from build123d import *

# Parameters (mm, degrees)
CHAMFER1_SIZE = 0.508


with BuildPart() as part:
    # Sketch1 → Revolve1 (revolve)
    with BuildSketch(Plane(origin=(0, 0, 0), x_dir=(0, 0, -1), z_dir=(1, 0, 0)), mode=Mode.PRIVATE) as revolve1_sk:
        Polygon((-85.5345, 19.05), (88.4465, 19.05), (88.4465, 25), (86.4145, 25), (86.4145, 23.5), (84.2645, 23.5), (84.2645, 25), (-84.2645, 25), (-84.2645, 25.4), (-85.5345, 25.4), align=None)
    revolve(revolve1_sk.sketch.rotate(Axis((0, 0, 0), (0, 0, 1)), 90), axis=Axis((0, 0, 0), (0, 0, 1)))

    # Chamfer1
    chamfer1_edges = [part.edges().sort_by_distance(p)[0] for p in [
        (25, 0, -88.4465),
    ]]
    chamfer(chamfer1_edges, length=CHAMFER1_SIZE)


solid = part.part
Part model, mm, in its own coordinate system. A direction names the side the tool comes from. Coordinates: 2 decimals unless noted, no trailing zeros. Order: outer loops, then holes, each group sorted by start corner. A loop starts at its lowest first (then second) coordinate and runs counter-clockwise, first axis right, second up. Notation, with made-up numbers: (-13.5, 45) - (24.5, 45) arc R14 ccw to (24.5, 50) - close; hole circle Ø4 at (16.5, -24.5). An arc over 180 degrees is marked (long way). Use CSV: the item, a comma, the result in double quotes.
Item 1: Saw through at C-C on z = -44.5. Give the cut face in (x, y).
Solved:
outline,"circle Ø50 at (0, 0); hole circle Ø38.1 at (0, 0)"
Item 2: Probe probe 1 along Y at (x, z) = (0, -53.5); probe 2 along X at (y, z) = (1, 66); probe 3 along Y at (x, z) = (-7.5, 28.5). List the from-to ranges inside material, lowest first.
Solved:
probe 1,"y = -25 to -19.05, 19.05 to 25"
probe 2,"x = -24.98 to -19.02, 19.02 to 24.98"
probe 3,"y = -23.85 to -17.51, 17.51 to 23.85"
Item 3: Mould opens along Z. For faces 1 (the face through (-17, 17, -84.264)), 2 (the face through (4.13, 18.597, -2.674)), 3 (the face through (-4, -19, 85.534)) say: +Z half, -Z half, draft (parallel to the pull), parting line (faces both ways), or undercut.
Solved:
face 1,"undercut"
face 2,"draft"
face 3,"+Z half"
Item 4: Drop flat-ended pins along their axis: P1, Ø8, axis at x = -14, z = -38.5, coming from the -Y side; P2, Ø2, axis at y = 1.5, z = -49, coming from the +X side (3 decimals); P3, Ø10, axis at y = -20, z = -11.5, coming from the +X side. Give the stop position or say it passes through.
Solved:
P1,"stops at y = -22.91"
P2,"stops at x = 24.995"
P3,"stops at x = 20"
Item 5: Saw through at A-A on x = 0. Give the cut face in (y, z), and give its area (3 significant figures).
Solved:
outline,"(-25.4, 84.26) - (-25, 84.26) - (-25, -84.26) - (-23.5, -84.26) - (-23.5, -86.41) - (-25, -86.41) - (-25, -87.94) - (-24.49, -88.45) - (-19.05, -88.45) - (-19.05, 85.53) - (-25.4, 85.53) - close; (19.05, -88.45) - (24.49, -88.45) - (25, -87.94) - (25, -86.41) - (23.5, -86.41) - (23.5, -84.26) - (25, -84.26) - (25, 84.26) - (25.4, 84.26) - (25.4, 85.53) - (19.05, 85.53) - close"
area,"2,060 mm²"
Item 6: 3-axis set-ups, long thin cutter, end or side, ignore diameter. For faces 4 (the face through (20.157, 15.456, 84.908)), 5 (the face through (-23.846, -7.509, 1.18)), 6 (the face through (17, 17, -86.414)): which of +Z, -Z, +X, -X, +Y, -Y reach the whole face in a straight line?
Solved:
face 4,"+Z, -Z"
face 5,"-Z"
face 6,"none"
